Check sheet for the modelled part. Datum: model origin and axes. Units: mm. Round coordinates to 2 decimals unless told otherwise and drop trailing zeros. Write each loop counter-clockwise with the first axis right and the second up, starting at its lowest first coordinate (ties: lowest second). Pieces come first, ordered by that corner, then holes.
Item 1: Section check B-B, the plane x = 173.8. Record the cut outline in (y, z), plus the area to 3 significant figures.
Item 2: Depth check by flat-ended pin: pin 1 (1 mm diameter, centred on x = 132.5, y = 0.5, fed in from -Z). Enter the tip coordinate at first touch or a pass-through.
Item 3: Section check A-A, the plane z = 3.2. Record the cut outline in (x, y), plus the area to 3 significant figures.
Item 4: Material ranges on line 1 along Z through (x, y) = (173.8, 0.45); line 2 along X through (y, z) = (1.1, 79.8); line 3 along X through (y, z) = (1.35, 79), recorded low to high.
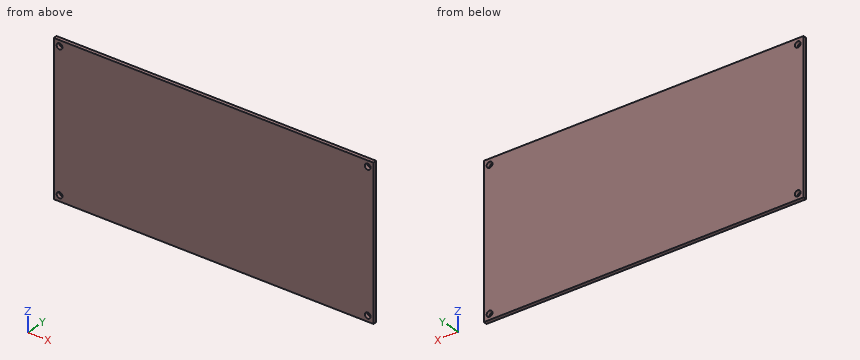
from build123d import *

# Parameters (mm, degrees)
ESQUISSE1_W             = 177
ESQUISSE1_H             = 83
BOSS_EXTRU_1_DEPTH      = 2
ENL_V_MAT_EXTRU_1_REACH = 197.504
ESQUISSE2_R             = 1.6


with BuildPart() as part:
    # Esquisse1 → Boss.-Extru.1 (new body)
    with BuildSketch(Plane(origin=(0, 0, 0), x_dir=(1, 0, 0), z_dir=(0, 1, 0))):
        with Locations((88.5, -41.5)):
            Rectangle(ESQUISSE1_W, ESQUISSE1_H)
    extrude(amount=BOSS_EXTRU_1_DEPTH)

    # Esquisse2 → Enlèv. mat.-Extru.1 (cut, up to next)
    with BuildSketch(Plane(origin=(0, 2, 0), x_dir=(1, 0, 0), z_dir=(0, 1, 0)), mode=Mode.PRIVATE) as enl_v_mat_extru_1_sk1:
        with Locations(Location((3.2, -3.2, 0), (0, 0, 270))):
            Circle(ESQUISSE2_R)
    enl_v_mat_extru_1_tool1 = extrude(enl_v_mat_extru_1_sk1.sketch, amount=-ENL_V_MAT_EXTRU_1_REACH, mode=Mode.PRIVATE) & part.part
    # Esquisse2 → Enlèv. mat.-Extru.1 (cut, up to next)
    with BuildSketch(Plane(origin=(0, 2, 0), x_dir=(1, 0, 0), z_dir=(0, 1, 0)), mode=Mode.PRIVATE) as enl_v_mat_extru_1_sk2:
        with Locations(Location((3.2, -79.8, 0), (0, 0, 270))):
            Circle(ESQUISSE2_R)
    enl_v_mat_extru_1_tool2 = extrude(enl_v_mat_extru_1_sk2.sketch, amount=-ENL_V_MAT_EXTRU_1_REACH, mode=Mode.PRIVATE) & part.part
    # Esquisse2 → Enlèv. mat.-Extru.1 (cut, up to next)
    with BuildSketch(Plane(origin=(0, 2, 0), x_dir=(1, 0, 0), z_dir=(0, 1, 0)), mode=Mode.PRIVATE) as enl_v_mat_extru_1_sk3:
        with Locations(Location((173.8, -3.2, 0), (0, 0, 270))):
            Circle(ESQUISSE2_R)
    enl_v_mat_extru_1_tool3 = extrude(enl_v_mat_extru_1_sk3.sketch, amount=-ENL_V_MAT_EXTRU_1_REACH, mode=Mode.PRIVATE) & part.part
    # Esquisse2 → Enlèv. mat.-Extru.1 (cut, up to next)
    with BuildSketch(Plane(origin=(0, 2, 0), x_dir=(1, 0, 0), z_dir=(0, 1, 0)), mode=Mode.PRIVATE) as enl_v_mat_extru_1_sk4:
        with Locations(Location((173.8, -79.8, 0), (0, 0, 270))):
            Circle(ESQUISSE2_R)
    enl_v_mat_extru_1_tool4 = extrude(enl_v_mat_extru_1_sk4.sketch, amount=-ENL_V_MAT_EXTRU_1_REACH, mode=Mode.PRIVATE) & part.part
    add(enl_v_mat_extru_1_tool1.solids().sort_by_distance((3.2, 2, 3.2))[0], mode=Mode.SUBTRACT)
    add(enl_v_mat_extru_1_tool2.solids().sort_by_distance((3.2, 2, 79.8))[0], mode=Mode.SUBTRACT)
    add(enl_v_mat_extru_1_tool3.solids().sort_by_distance((173.8, 2, 3.2))[0], mode=Mode.SUBTRACT)
    add(enl_v_mat_extru_1_tool4.solids().sort_by_distance((173.8, 2, 79.8))[0], mode=Mode.SUBTRACT)


solid = part.part
Values found:
1. outline: (0, 0) - (2, 0) - (2, 1.6) - (0, 1.6) - close; (0, 4.8) - (2, 4.8) - (2, 78.2) - (0, 78.2) - close; (0, 81.4) - (2, 81.4) - (2, 83) - (0, 83) - close
1. area: 153 mm2
2. pin 1: stops at z = 0
3. outline: (0, 0) - (1.6, 0) - (1.6, 2) - (0, 2) - close; (4.8, 0) - (172.2, 0) - (172.2, 2) - (4.8, 2) - close; (175.4, 0) - (177, 0) - (177, 2) - (175.4, 2) - close
3. area: 341 mm2
4. line 1: z = 0 to 1.6, 4.8 to 78.2, 81.4 to 83
4. line 2: x = 0 to 1.6, 4.8 to 172.2, 175.4 to 177
4. line 3: x = 0 to 1.81, 4.59 to 172.41, 175.19 to 177
